Verification items for the finished model (mm, model axes). A direction names the side the tool comes from. Round coordinates to 2 decimals unless told otherwise and drop trailing zeros. Write each loop counter-clockwise with the first axis right and the second up, starting at its lowest first coordinate (ties: lowest second). Pieces come first, ordered by that corner, then holes. Notation, with made-up numbers: (-13, 83) - (26, 83) arc R27 ccw to (26, 102) - close; hole circle Ø4 at (-6.75, 2). An arc over 180 degrees is marked (long way). Answer as a JSON object with one key per item and string values. Group by question number.
1) Thickness scan on line 1 (X direction, y = -0.5, z = 17.75); line 2 (Y direction, x = 8, z = 17.75); line 3 (X direction, y = 2.5, z = 18.5). Record the ranges inside material, lowest first.
2) Section check A-A (x = -27). Enter the section's corners in (y, z).
3) Mould release check, pull along X, two halves, no side actions. Record for faces 1 (the flat face through (11, 3.106, 12)), 2 (the flat face through (-5, 0, 25)): +X half, -X half, draft (parallel to the pull), parting line (faces both ways), or undercut.
4) Section check C-C (y = 12). Enter the section's corners in (x, z).
5) Go/stop test with flat-tipped pins: pin 1 Ø6 at (x, z) = (-28, 13) entering from +Y; pin 2 Ø4 at (x, z) = (-15, 8.5) entering from -Y; pin 3 Ø1 at (y, z) = (1, 6.5) entering from -X. Record where each tip stops, or that it passes through.
6) Section check B-B (z = 16.5). Enter the section's corners in (x, y), then the cut area to 3 significant figures.
7) Set-up check for faces 3 (the cylindrical face through (30.221, 3.673, 12.325)), 4 (the flat face through (36.081, 0, 12)), 5 (the flat face through (-5, 0, 0)), 6 (the flat face through (11, -7.911, 12)): record each of +Z, -Z, +X, -X, +Y, -Y from which the full face is reachable in a straight line by a thin tool's end or side.
```python
from build123d import *

# Parameters (mm, degrees)
F1_DEPTH = 25


with BuildPart() as f1:
    # F0 (on Top) → F1 (new body)
    with BuildSketch(Plane.XY):
        with BuildLine():
            ThreePointArc((37.7576954416, -9.2102163582), (47.7291677906, -8.725438733), (52.5801459464, 0))
            ThreePointArc((52.5801459464, 0), (45.0359965694, 9.9037039133), (33.4842184117, 5.2610793948))
            ThreePointArc((33.4842184117, 5.2610793948), (32.1020667525, -1.1741087466), (34.9094763525, -7.1272962089))
            ThreePointArc((34.9094763525, -7.1272962089), (36.4520652966, -8.0067456142), (37.7576954416, -9.2102163582))
        make_face()
        Polygon((46.0107769178, 5.4953820164), (50.0034056604, 0), (44.6856294577, -7.3192910224), (36.0812868173, -4.5235706254), (36.0812868173, 4.5235706254), (44.6856294577, 7.3192910224), align=None, mode=Mode.SUBTRACT)
        with BuildLine():
            ThreePointArc((34.9094763525, -7.1272962089), (32.1020667525, -1.1741087466), (33.4842184117, 5.2610793948))
            ThreePointArc((33.4842184117, 5.2610793948), (30.1721208062, 3.6571952775), (26.53361631, 3.1060874462))
            Line((26.53361631, 3.1060874462), (-4.9357796088, 3.1060874462))
            ThreePointArc((-4.9357796088, 3.1060874462), (-8.0929029993, 3.2954334717), (-10.29699962, 5.5637452022))
            ThreePointArc((-10.29699962, 5.5637452022), (-9.5238230465, 2.8294901369), (-9.2631732017, 0))
            ThreePointArc((-9.2631732017, 0), (-9.8138730709, -4.0933289992), (-11.4268110085, -7.8955709497))
            ThreePointArc((-11.4268110085, -7.8955709497), (-8.1795839214, -7.1670230809), (-4.9357796088, -7.9106623307))
            Line((-4.9357796088, -7.9106623307), (27.3132491857, -7.9106623307))
            ThreePointArc((27.3132491857, -7.9106623307), (31.0097542861, -6.533691424), (34.9094763525, -7.1272962089))
        make_face()
        with BuildLine():
            ThreePointArc((4.0779244155, -4.9060937017), (1.0056323331, -2.7925497007), (3.4770111088, 0))
            Line((3.4770111088, 0), (20.5028969795, 0))
            ThreePointArc((20.5028969795, 0), (22.9641081907, -2.6703736104), (20.102288574, -4.9060937017))
            Line((20.102288574, -4.9060937017), (4.0779244155, -4.9060937017))
        make_face(mode=Mode.SUBTRACT)
        with BuildLine():
            ThreePointArc((34.9094763525, -7.1272962089), (36.2434833253, -8.2919640144), (37.7576954416, -9.2102163582))
            ThreePointArc((37.7576954416, -9.2102163582), (36.4520652966, -8.0067456142), (34.9094763525, -7.1272962089))
        make_face()
        with BuildLine():
            ThreePointArc((-10.3811004349, 5.7774928533), (-10.3404533777, 5.6700668678), (-10.29699962, 5.5637452022))
            ThreePointArc((-10.29699962, 5.5637452022), (-10.3386537721, 5.6707749377), (-10.3811004349, 5.7774928533))
        make_face()
        with BuildLine():
            ThreePointArc((-9.2631732017, 0), (-9.5238230465, 2.8294901369), (-10.29699962, 5.5637452022))
            ThreePointArc((-10.29699962, 5.5637452022), (-10.3404533777, 5.6700668678), (-10.3811004349, 5.7774928533))
            ThreePointArc((-10.3811004349, 5.7774928533), (-40.1943173282, 1.1810763551), (-11.4268110085, -7.8955709497))
            ThreePointArc((-11.4268110085, -7.8955709497), (-9.8138730709, -4.0933289992), (-9.2631732017, 0))
        make_face()
        Polygon((-19.7663526565, 8.9728942857), (-14.4880691335, 0.1693609529), (-19.4730108813, -8.8035333329), (-29.7362361521, -8.9728942857), (-35.0145196751, -0.1693609529), (-30.0295779273, 8.8035333329), align=None, mode=Mode.SUBTRACT)
    extrude(amount=F1_DEPTH)


solid = f1.part
```
Returned:
{
 "1": {"line 1": "-40.23 to -34.82, -14.86 to 1.98, 21.99 to 36.08, 49.64 to 52.57", "line 2": "-7.91 to -4.91, 0 to 3.11", "line 3": "-40.04 to -33.53, -15.89 to 36.08, 48.19 to 52.27"},
 "2": {"outline": "(-15.32, 0) - (-8.93, 0) - (-8.93, 25) - (-15.32, 25) - close; (8.85, 0) - (15.32, 0) - (15.32, 25) - (8.85, 25) - close"},
 "3": {"face 1": "undercut", "face 2": "draft"},
 "4": {"outline": "(-34.54, 0) - (-14.96, 0) - (-14.96, 25) - (-34.54, 25) - close"},
 "5": {"pin 1": "y = 15.49", "pin 2": "y = -13.41", "pin 3": "x = -40.23"},
 "6": {"outline": "(-11.43, -7.9) arc R7.52 cw to (-4.94, -7.91) - (27.31, -7.91) arc R7.85 cw to (34.91, -7.13) arc R10.27 ccw (long way) to (33.48, 5.26) arc R12.29 cw to (26.53, 3.11) - (-4.94, 3.11) arc R4.37 cw to (-10.3, 5.56) arc R15.49 ccw (long way) to start; hole (-35.01, -0.17) - (-29.74, -8.97) - (-19.47, -8.8) - (-14.49, 0.17) - (-19.77, 8.97) - (-30.03, 8.8) - close; hole (3.48, 0) arc R2.49 ccw (long way) to (4.08, -4.91) - (20.1, -4.91) arc R2.47 ccw (long way) to (20.5, 0) - close; hole (36.08, -4.52) - (44.69, -7.32) - (50, 0) - (44.69, 7.32) - (36.08, 4.52) - close", "area": "1,030 mm2"},
 "7": {"face 3": "+Z, -Z, +Y", "face 4": "+Z, -Z", "face 5": "-Z, +X, -X, +Y, -Y", "face 6": "+Z, -Z, -Y"}
}
